Part print with two shaded views. Sizes in mm from the minimum x, y, z corner. Give positions to 0.01 mm unless a question says otherwise; leave off trailing zeros. Write each loop counter-clockwise with the first axis right and the second up, starting at its lowest first coordinate (ties: lowest second). Pieces come first, ordered by that corner, then holes.
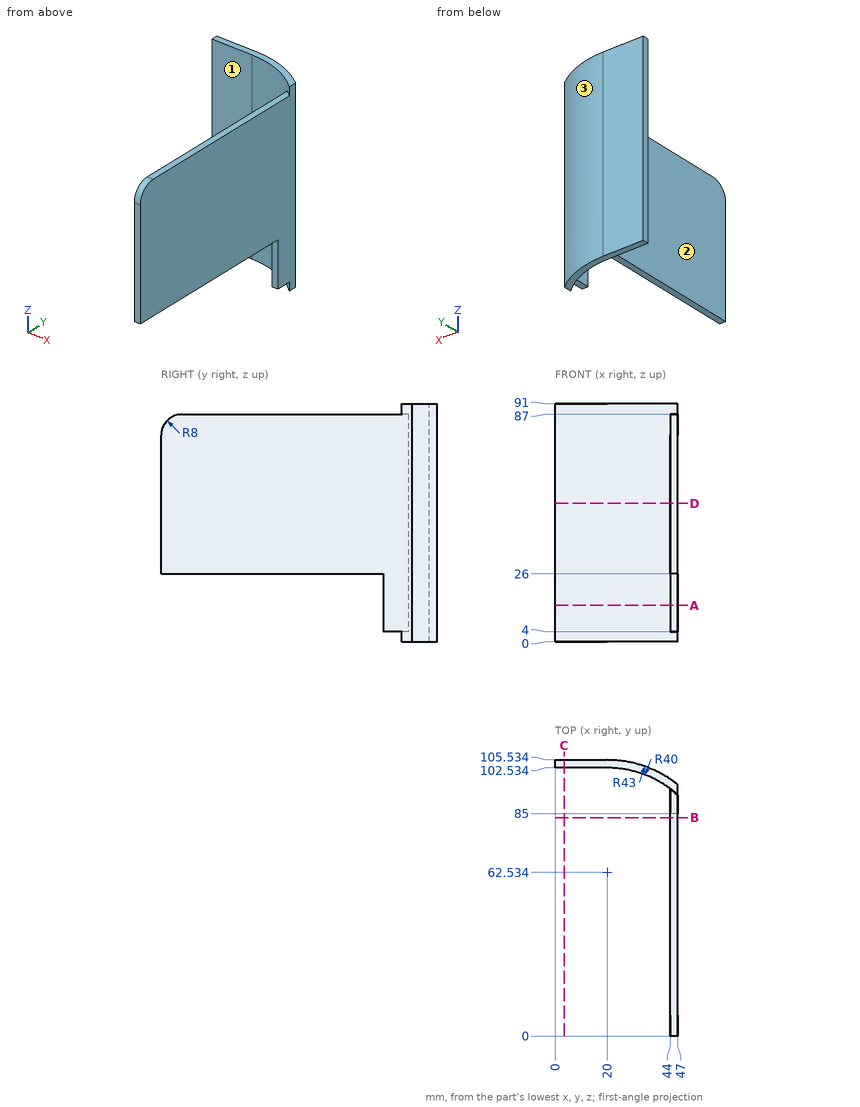
1) Saw through at D-D, the plane z = 53. Write the cut outline in (x, y).
Answers follow:
outline: (0, 102.53) - (20, 102.53) arc R40 cw to (44, 94.53) - (44, 0) - (47, 0) - (47, 96) arc R43 ccw to (20, 105.53) - (0, 105.53) - close
2) Two-plate mould, pull along Y, no slides. Class the marked faces 1, 2 and 3: +Y half, -Y half, draft (parallel to the pull), parting line (faces both ways), or undercut.
Answers follow:
face 1: -Y half
face 2: draft
face 3: +Y half
3) Pin check, flat tips, straight feed: pin 1 Ø3.5 at (x, y) = (45.5, 43) entering from -Z; pin 2 Ø1.5 at (x, y) = (45.5, 39.5) entering from +Z; pin 3 Ø6 at (y, z) = (90, 58.5) entering from -X. Stop position of each tip, or through.
Answers follow:
pin 1: stops at z = 26
pin 2: stops at z = 87
pin 3: stops at x = 44
4) Wall check: L1, parallel to Y at x = 15, z = 12.5; L2, parallel to X at y = 48.5, z = 48; L3, parallel to Z at x = 45, y = 73.5. Give the ranges that are in metal, low to high.
Answers follow:
L1: y = 102.53 to 105.53
L2: x = 44 to 47
L3: z = 26 to 87
5) Saw through at B-B, the plane y = 83.5. Write the cut outline in (x, z).
Answers follow:
outline: (44, 26) - (47, 26) - (47, 87) - (44, 87) - close
6) Saw through at C-C, the plane x = 3.5. Write the cut outline in (y, z), then the cut area to 3 significant figures.
Answers follow:
outline: (102.53, 0) - (105.53, 0) - (105.53, 91) - (102.53, 91) - close
area: 273 mm2
7) Saw through at A-A, the plane z = 14. Write the cut outline in (x, y), then the cut area to 3 significant figures.
Answers follow:
outline: (0, 102.53) - (20, 102.53) arc R40 cw to (44, 94.53) - (44, 85) - (47, 85) - (47, 96) arc R43 ccw to (20, 105.53) - (0, 105.53) - close
area: 173 mm2
